from build123d import *

# Parameters (mm, degrees)
SKETCH1_W                = 86.52
SKETCH1_H                = 65
BOSS_EXTRUDE1_DEPTH      = 1.2
SKETCH2_W                = 66
SKETCH2_H                = 1
BOSS_EXTRUDE2_DEPTH      = 65
BOSS_EXTRUDE5_DEPTH      = 3
BOSS_EXTRUDE5_DEPTH_BACK = 0.01
CHAMFER1_SIZE            = 2
CHAMFER2_SIZE            = 2
CHAMFER3_SIZE            = 1
SKETCH5_W                = 2.3
SKETCH5_H                = 1.199074312
BOSS_EXTRUDE7_DEPTH      = 8
CHAMFER5_SIZE            = 0.5
FILLET3_R                = 0.5


with BuildPart() as part:
    # Sketch1 → Boss-Extrude1 (new body)
    with BuildSketch(Plane(origin=(0, 0, 0), x_dir=(1, 0, 0), z_dir=(0, 1, 0))):
        Rectangle(SKETCH1_W, SKETCH1_H)
    extrude(amount=BOSS_EXTRUDE1_DEPTH)

    # Sketch2 → Boss-Extrude2 (add)
    with BuildSketch(Plane.XY.offset(32.5)):
        with Locations((0, 1.7)):
            Rectangle(SKETCH2_W, SKETCH2_H)
    extrude(amount=-BOSS_EXTRUDE2_DEPTH)

    # Sketch3 → Boss-Extrude5 (add, two sides: drawn at the far end of the back side and taken through both)
    with BuildSketch(Plane(origin=(0, 0, -32.5), x_dir=(-1, 0, 0), z_dir=(0, 0, -1)).offset(-BOSS_EXTRUDE5_DEPTH_BACK)):
        Polygon((-43.26, 1.2), (-43.26, 1.199074312), (-50.859139548, 1.199074312), (-50.859139548, 0), (-40.26, 0), (-40.26, 1.2), align=None)
        Polygon((40.26, 1.2), (40.26, 0), (50.859139548, 0), (50.859139548, 1.199074312), (43.26, 1.199074312), (43.26, 1.2), align=None)
    extrude(amount=BOSS_EXTRUDE5_DEPTH + BOSS_EXTRUDE5_DEPTH_BACK)

    # Chamfer1
    chamfer1_edges = [part.edges().sort_by_distance(p)[0] for p in [
        (40.26, 0.6, -35.5),
    ]]
    chamfer(chamfer1_edges, length=CHAMFER1_SIZE)

    # Chamfer2
    chamfer2_edges = [part.edges().sort_by_distance(p)[0] for p in [
        (-40.26, 0.6, -35.5),
    ]]
    chamfer(chamfer2_edges, length=CHAMFER2_SIZE)

    # Chamfer3
    chamfer3_edges = [part.edges().sort_by_distance(p)[0] for p in [
        (-40.26, 0.6, -32.5),
        (40.26, 0.6, -32.5),
    ]]
    chamfer(chamfer3_edges, length=CHAMFER3_SIZE - 0.0001)  # a hair under: the kernel refuses the full size

    # Sketch5 → Boss-Extrude7 (add)
    with BuildSketch(Plane.XY.offset(-32.49)):
        with Locations((-49.709139548, 0.599537156)):
            Rectangle(SKETCH5_W, SKETCH5_H)
        with Locations((49.709139548, 0.599537156)):
            Rectangle(SKETCH5_W, SKETCH5_H)
    extrude(amount=BOSS_EXTRUDE7_DEPTH)

    # Chamfer5
    chamfer5_edges = [part.edges().sort_by_distance(p)[0] for p in [
        (-48.559139548, 0.599537156, -24.49),
        (-50.859139548, 0.599537156, -24.49),
        (50.859139548, 0.599537156, -24.49),
        (48.559139548, 0.599537156, -24.49),
        (-50.859139548, 0.599537156, -35.5),
        (50.859139548, 0.599537156, -35.5),
    ]]
    chamfer(chamfer5_edges, length=CHAMFER5_SIZE)

    # Fillet3
    fillet3_edges = [part.edges().sort_by_distance(p)[0] for p in [
        (-48.559139548, 0.599537156, -32.49),
        (48.559139548, 0.599537156, -32.49),
        (-43.26, 0.599537156, -32.49),
        (43.26, 0.599537156, -32.49),
    ]]
    fillet(fillet3_edges, radius=FILLET3_R)


solid = part.part
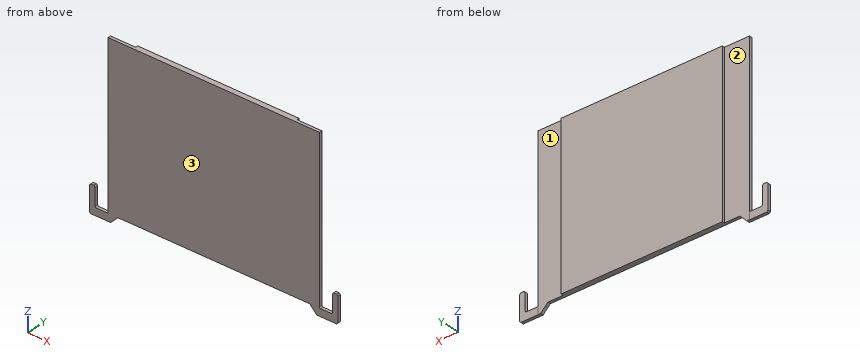
Check sheet for the modelled part. Datum: model origin and axes. Units: mm. Face numbers are marked on the shaded views. A direction names the side the tool comes from. Round coordinates to 2 decimals unless told otherwise and drop trailing zeros. Loops run counter-clockwise (first coordinate to the right, second up) from the corner with the lowest first, then second, coordinate; pieces in that order, holes last. Notation, with made-up numbers: M 89.5,25 L 145.5,25 A21 ccw 145.5,62 Z; hole C 84,81.25 d7. An arc over 180 degrees is marked long. One line per item, written item: value.
(1) Access from +Z, -Z, +X, -X, +Y, -Y to the whole of each face (thin tool, end or side, straight path). Record for the marked faces 1, 2 and 3.
Computed values:
face 1: +Z, -Z, +X, +Y
face 2: +Z, -Z, -X, +Y
face 3: +Z, -Z, +X, -X, -Y
(2) Sectioned sample at A-A, the plane z = -28.5. Record the cut outline in (x, y), then the cut area to 3 significant figures.
Computed values:
outline: M -50.86,0 L -48.56,0 L -48.56,1.2 L -50.86,1.2 Z; M -43.26,0 L 43.26,0 L 43.26,1.2 L 33,1.2 L 33,2.2 L -33,2.2 L -33,1.2 L -43.26,1.2 Z; M 48.56,0 L 50.86,0 L 50.86,1.2 L 48.56,1.2 Z
area: 175 mm^2
(3) Sectioned sample at C-C, the plane z = -1.5. Record the cut outline in (x, y).
Computed values:
outline: M -43.26,0 L 43.26,0 L 43.26,1.2 L 33,1.2 L 33,2.2 L -33,2.2 L -33,1.2 L -43.26,1.2 Z
(4) Thickness scan on line 1 (X direction, y = 0.3, z = 23.5); line 2 (X direction, y = 1.5, z = 10); line 3 (Y direction, x = 42.5, z = -18). Record the ranges inside material, lowest first.
Computed values:
line 1: x = -43.26 to 43.26
line 2: x = -33 to 33
line 3: y = 0 to 1.2
(5) Sectioned sample at D-D, the plane x = -13. Record the cut outline in (y, z).
Computed values:
outline: M 0,-32.5 L 2.2,-32.5 L 2.2,32.5 L 0,32.5 Z
(6) Depth check by flat-ended pin: pin 1 Ø2.5 at (x, z) = (-48.5, -32.5) entering from +Y; pin 2 Ø1 at (y, z) = (0.5, 14) entering from -X; pin 3 Ø1 at (x, y) = (46.5, 0.5) entering from +Z; pin 4 Ø2.5 at (x, z) = (45, -30.5) entering from +Y. Enter the tip coordinate at first touch or a pass-through.
Computed values:
pin 1: stops at y = 1.2
pin 2: stops at x = -43.26
pin 3: stops at z = -32.49
pin 4: passes through
